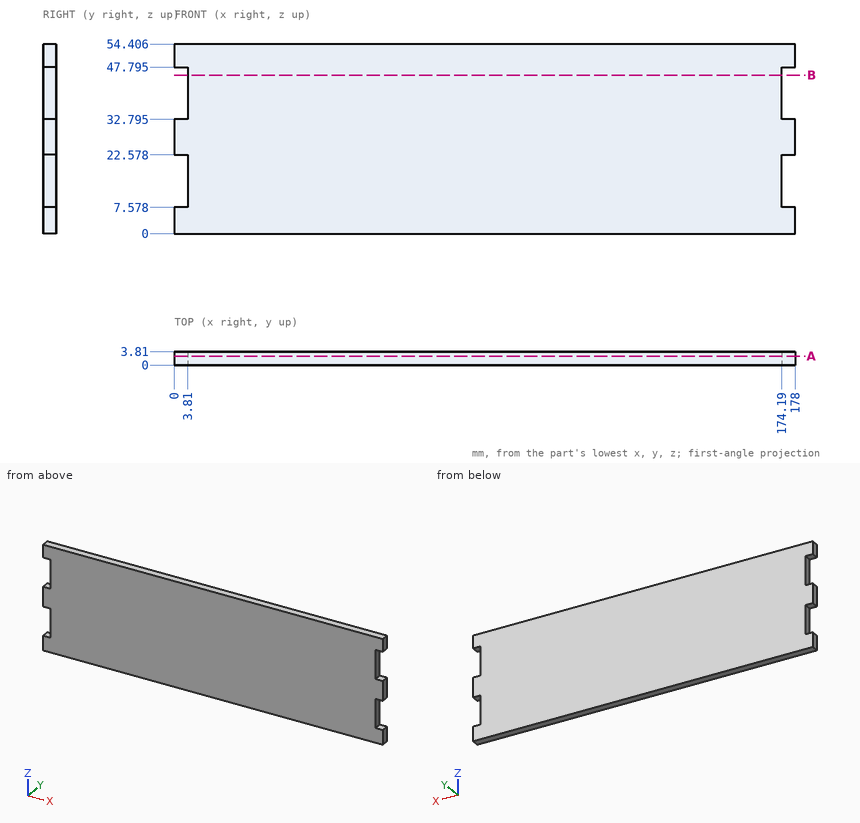
Part print with two shaded views. Sizes in mm from the minimum x, y, z corner. Round coordinates to 2 decimals unless told otherwise and drop trailing zeros. Order: outer loops, then holes, each group sorted by start corner. A loop starts at its lowest first (then second) coordinate and runs counter-clockwise, first axis right, second up. Notation, with made-up numbers: (-2, 51) - (2, 51) arc R28 ccw to (2, 79) - close; hole circle Ø6 at (80.25, 9). An arc over 180 degrees is marked (long way). Answer in a Markdown table with one row per item. Add a question column.
(1) Band-saw the part on B-B on z = 45.5. List the corners of the cut face in (x, y).
(2) Probe L1, parallel to X at y = 3.4, z = 46.5. List the from-to ranges inside material, lowest first. Write a range as [from, to].
(3) Band-saw the part on A-A on y = 2.55. List the corners of the cut face in (x, z) (1 decimal).
(4) Drop flat-ended pins along their axis: pin 1 Ø1.1 at (y, z) = (2.5, 16) entering from +X; pin 2 Ø1.1 at (y, z) = (1, 39.5) entering from -X. Give the stop position or say it passes through.
Data:
| question | item | result |
|---|---|---|
| 1 | outline | (3.81, 0) - (174.19, 0) - (174.19, 3.81) - (3.81, 3.81) - close |
| 2 | L1 | x = [3.81, 174.19] |
| 3 | outline | (0, 0) - (178, 0) - (178, 7.6) - (174.2, 7.6) - (174.2, 22.6) - (178, 22.6) - (178, 32.8) - (174.2, 32.8) - (174.2, 47.8) - (178, 47.8) - (178, 54.4) - (0, 54.4) - (0, 47.8) - (3.8, 47.8) - (3.8, 32.8) - (0, 32.8) - (0, 22.6) - (3.8, 22.6) - (3.8, 7.6) - (0, 7.6) - close |
| 4 | pin 1 | stops at x = 174.19 |
| 4 | pin 2 | stops at x = 3.81 |
